Input: part model. Units: mm. Frame: model coordinates. A direction names the side the tool comes from. Coordinates: 2 decimals unless noted, no trailing zeros. Order: outer loops, then holes, each group sorted by start corner. A loop starts at its lowest first (then second) coordinate and runs counter-clockwise, first axis right, second up. Notation, with made-up numbers: M -22.5,57.5 L -15.5,57.5 A15 cw -15.5,67.5 Z; hole C -11.75,-31.5 d4. An arc over 180 degrees is marked long. Answer in a Markdown table with one row per item.
from build123d import *

# Parameters (mm, degrees)
F0_W     = 38.1
F0_H     = 38.1
F1_DEPTH = 38.1
F5_DEPTH = 38.1
F7_DEPTH = 38.1
F8_W     = 25.4
F8_H     = 7.62
F9_DEPTH = 38.1


with BuildPart() as f1:
    # F0 (on Front) → F1 (new body)
    with BuildSketch(Plane.XZ):
        with Locations((19.05, 19.05)):
            Rectangle(F0_W, F0_H)
    extrude(amount=F1_DEPTH)

    # F4 (on Front) → F5 (cut)
    with BuildSketch(Plane.XZ):
        Polygon((6.35, 0), (0, 38.1), (0, 0), align=None)
        Polygon((31.75, 38.1), (6.35, 38.1), (11.43, 15.875), (16.51, 28.575), (21.59, 28.575), (26.67, 15.875), align=None)
        Polygon((19.05, 15.875), (12.7, 0), (25.4, 0), align=None)
        Polygon((38.1, 0), (38.1, 38.1), (31.75, 0), align=None)
    extrude(amount=F5_DEPTH, mode=Mode.SUBTRACT)

    # F6 (on offset) → F7 (cut)
    with BuildSketch(Plane.YZ.offset(38.1)):
        Polygon((-38.1, 38.1), (-38.1, 0), (-31.75, 38.1), align=None)
        Polygon((-19.05, 22.225), (-12.7, 38.1), (-25.4, 38.1), align=None)
        Polygon((-31.75, 0), (-7.027086, 0), (-11.43, 22.225), (-16.51, 10.050542), (-21.59, 10.050542), (-26.67, 22.225), align=None)
        Polygon((-6.35, 38.1), (0, 0), (0, 38.1), align=None)
    extrude(amount=-F7_DEPTH, mode=Mode.SUBTRACT)

    # F8 (on offset) → F9 (cut)
    with BuildSketch(Plane.XY.offset(38.1)):
        with Locations((12.7, -26.67)):
            Rectangle(F8_W, F8_H)
        with Locations((25.4, -11.43)):
            Rectangle(F8_W, F8_H)
    extrude(amount=-F9_DEPTH, mode=Mode.SUBTRACT)


solid = f1.part
1) Cut plane A-A, the plane z = 29.5. Output: boundary loops of the cut face in (x, y), and give its area (3 significant figures).
Resolved:
| item | result |
|---|---|
| outline | M 1.43,-33.18 L 8.32,-33.18 L 8.32,-30.48 L 1.43,-30.48 Z; M 1.43,-22.86 L 8.32,-22.86 L 8.32,-21.96 L 1.43,-21.96 Z; M 1.43,-16.14 L 8.32,-16.14 L 8.32,-4.92 L 1.43,-4.92 Z; M 29.78,-33.18 L 36.67,-33.18 L 36.67,-21.96 L 29.78,-21.96 Z; M 29.78,-16.14 L 36.67,-16.14 L 36.67,-15.24 L 29.78,-15.24 Z; M 29.78,-7.62 L 36.67,-7.62 L 36.67,-4.92 L 29.78,-4.92 Z |
| area | 204 mm2 |
2) Cut plane B-B, the plane x = 27.5. Output: boundary loops of the cut face in (y, z), and give its area (3 significant figures).
Resolved:
| item | result |
|---|---|
| outline | M -38.1,0 L -31.75,0 L -27.29,19.51 L -34.85,19.51 Z; M -25.54,19.51 L -21.59,10.05 L -16.51,10.05 L -15.24,13.09 L -15.24,19.51 Z; M -7.62,2.99 L -7.03,0 L 0,0 L -3.25,19.51 L -7.62,19.51 Z |
| area | 328 mm2 |
3) Cut plane D-D, the plane y = -34.5. Output: boundary loops of the cut face in (x, z) (3 decimals).
Resolved:
| item | result |
|---|---|
| outline | M 2.75,21.6 L 6.35,0 L 12.7,0 L 19.05,15.875 L 25.4,0 L 31.75,0 L 35.35,21.6 L 27.979,21.6 L 26.67,15.875 L 24.38,21.6 L 13.72,21.6 L 11.43,15.875 L 10.121,21.6 Z |
4) Reachability of faces 1 (the face through (28.61, -25.21, 24.36)), 2 (the face through (5.6, -21, 27.1)), 3 (the face through (25, -7.62, 17)) from +Z, -Z, +X, -X, +Y, -Y: full face, straight path, thin tool, end or side. Return the list, or none.
Resolved:
| item | result |
|---|---|
| face 1 | +Z, +Y, -Y |
| face 2 | +Z, +X, -X |
| face 3 | +Z, -Z, +X |
5) Contact query for flat-ended pins moving along their axis: pin 1 (1 mm diameter, centred on x = 20, y = -22.5, fed in from +Z) (3 decimals); pin 2 (2 mm diameter, centred on y = -14.5, z = 16, fed in from +X); pin 3 (2.5 mm diameter, centred on y = -28.5, z = 11, fed in from -X); pin 4 (12 mm diameter, centred on x = 15, y = -29.5, fed in from -Z). Output: stop coordinate, or through.
Resolved:
| item | result |
|---|---|
| pin 1 | stops at z = 28.575 |
| pin 2 | stops at x = 34.53 |
| pin 3 | stops at x = 25.4 |
| pin 4 | stops at z = 0 |
6) Mould query, pull axis Y, two halves, no side actions, for faces 4 (the face through (22.27, -33.39, 7.83)), 5 (the face through (19.32, -34.97, 18.78)), 6 (the face through (27, -19, 10.051)). Classes: +Y half, -Y half, draft (parallel to the pull), parting line (faces both ways), or undercut.
Resolved:
| item | result |
|---|---|
| face 4 | draft |
| face 5 | -Y half |
| face 6 | undercut |
7) Material intervals for probe 1 along Y at (x, z) = (8, 14); probe 2 along Y at (x, z) = (21, 16); probe 3 along X at (y, z) = (-16, 22), sorted ascending.
Resolved:
| item | result |
|---|---|
| probe 1 | y = -35.77 to -30.48, -22.86 to -14.86, -9.8 to -2.33 |
| probe 2 | y = -35.43 to -30.48, -22.86 to -15.24, -7.62 to -2.67 |
| probe 3 | x = 2.68 to 10.03, 13.88 to 24.22, 28.07 to 35.42 |
